Read the model definition and answer for the solid it produces. Units are mm, in the model's axes. Give positions to 0.01 mm unless a question says otherwise; leave off trailing zeros. Order: outer loops, then holes, each group sorted by start corner. A loop starts at its lowest first (then second) coordinate and runs counter-clockwise, first axis right, second up. Notation, with made-up numbers: M 13.5,66.5 L 65.5,66.5 A19 ccw 65.5,79.5 Z; hole C -25,51 d5. An arc over 180 degrees is marked long. Write item = value, one per line. Start each with the question number.
from build123d import *

# Parameters (mm, degrees)
BOSS_EXTRUDE1_DEPTH = 2.9
CUT_EXTRUDE1_REACH  = 4.9
SKETCH2_R           = 1.85


with BuildPart() as part:
    # Sketch1 → Boss-Extrude1 (new body)
    with BuildSketch(Plane(origin=(0, 0, 0), x_dir=(1, 0, 0), z_dir=(0, 1, 0))):
        Polygon((0, 3.868246804), (-3.35, 1.934123402), (-3.35, -1.934123402), (0, -3.868246804), (3.35, -1.934123402), (3.35, 1.934123402), align=None)
    extrude(amount=BOSS_EXTRUDE1_DEPTH)

    # Sketch2 → Cut-Extrude1 (cut, up to next)
    with BuildSketch(Plane(origin=(0, 2.9, 0), x_dir=(1, 0, 0), z_dir=(0, 1, 0)), mode=Mode.PRIVATE) as cut_extrude1_sk1:
        Circle(SKETCH2_R)
    cut_extrude1_tool1 = extrude(cut_extrude1_sk1.sketch, amount=-CUT_EXTRUDE1_REACH, mode=Mode.PRIVATE) & part.part
    add(cut_extrude1_tool1.solids().sort_by_distance((0, 2.9, 0))[0], mode=Mode.SUBTRACT)


solid = part.part
1) Find the intervals of material crossed by probe 1 along X at (y, z) = (0.95, 0); probe 2 along X at (y, z) = (1.15, -2.75); probe 3 along Z at (x, y) = (0.75, 0.6), in increasing order. Write a range as [from, to].
2) Find section C-C on x = -1. Determine the outline of the cut face in (y, z).
3) This flat-tipped pin is pushed along its axis until it touches: P1, Ø1, axis at x = 2.5, y = 2.5, coming from the -Z side. Where does it stop, or does it pass through?
4) Find section A-A on y = 1.5. Determine the outline of the cut face in (x, z), plus the area to 3 significant figures.
5) Find section B-B on x = -0.25. Determine the outline of the cut face in (y, z), plus the area to 3 significant figures.
6) Find section D-D on z = 3.25. Determine the outline of the cut face in (x, y).
7) For a pull along X with two mould halves and no side action, classify faces 1 (the face through (-1, 2.9, -2)), 2 (the face through (-3.35, 1, 0)), 3 (the face through (-0.401, 1.47, 1.806)), 4 (the face through (3.35, 1, 0)) as pulls with the +X half, pulls with the -X half, needs draft (parallel to the pull), parting line crosses it, or undercut.
Numbers:
q1.probe_1 = [-3.35, -1.85], [1.85, 3.35]
q1.probe_2 = [-1.94, 1.94]
q1.probe_3 = [-3.44, -1.69], [1.69, 3.44]
q2.outline = M 0,-3.29 L 2.9,-3.29 L 2.9,-1.56 L 0,-1.56 Z; M 0,1.56 L 2.9,1.56 L 2.9,3.29 L 0,3.29 Z
q3.P1 = -2.71
q4.outline = M -3.35,-1.93 L 0,-3.87 L 3.35,-1.93 L 3.35,1.93 L 0,3.87 L -3.35,1.93 Z; hole C 0,0 d3.7
q4.area = 28.1 mm2
q5.outline = M 0,-3.72 L 2.9,-3.72 L 2.9,-1.83 L 0,-1.83 Z; M 0,1.83 L 2.9,1.83 L 2.9,3.72 L 0,3.72 Z
q5.area = 11.0 mm2
q6.outline = M -1.07,0 L 1.07,0 L 1.07,2.9 L -1.07,2.9 Z
q7.face_1 = needs draft
q7.face_2 = pulls with the -X half
q7.face_3 = undercut
q7.face_4 = pulls with the +X half
